Autodesk Inventor part; units mm, degrees
ref_plane "YZ Plane" through (0, 0, 0) normal (1, 0, 0) x (0, 1, 0)
ref_plane "XZ Plane" through (0, 0, 0) normal (0, 1, 0) x (-1, 0, 0)
ref_plane "XY Plane" through (0, 0, 0) normal (0, 0, 1) x (1, 0, 0)
sketch "Sketch1" plane through (0, 0, 0) normal (0, 1, 0) x (-1, 0, 0)
  circle A0 centre (0, 0) radius 165
  circle A1 centre (0, 0) radius 175
  line L0 (0, 0) -> (175, 0)
  line L1 (0, 0) -> (169.037, -45.2933)
  point P0 (159.3778, -42.7051)
  point P1 (165, 0)
  dimension "d0" = 10
  dimension "d1" = 330
  dimension "d2" = 15
extrude "Extrusion1" add sketch "Sketch1" along normal blind 5 contours L0 A1 L1 A0 picked at (171.4447, -5.0841)
sketch "Sketch3" plane through (0, 5, 0) normal (0, 1, 0) x (1, 0, 0)
  arc A0 (-169.037, 45.2933) -> (-175, 0) centre (0, 0) ccw
  line L0 (-175, 0) -> (-165, 0)
  arc A1 (-159.3778, 42.7051) -> (-165, 0) centre (0, 0) ccw
  line L1 (-159.3778, 42.7051) -> (-169.037, 45.2933)
  circle A2 centre (0, 0) radius 175
  circle A3 centre (0, 0) radius 165
  circle A4 centre (0, 0) radius 195
  line L2 (0, 0) -> (-188.3555, 50.4697)
  line L3 (0, 0) -> (-195, 0)
  point P0 (-175, 0)
  dimension "d10" = 20
extrude "Extrusion2" add sketch "Sketch3" along normal blind 10 contours L1 A1 L0 A0 | A0 L3 A4 L2
sketch "Sketch4" plane through (0, 0, 0) normal (0, -1, 0) x (1, 0, 0)
  arc A0 (-195, 0) -> (-188.3555, -50.4697) centre (0, 0) ccw
  arc A1 (-175, 0) -> (-169.037, -45.2933) centre (0, 0) ccw
  line L0 (-159.3778, -42.7051) -> (-169.037, -45.2933)
  arc A2 (-165, 0) -> (-159.3778, -42.7051) centre (0, 0) ccw
  line L1 (-175, 0) -> (-165, 0)
  circle A3 centre (0, 0) radius 175
  circle A4 centre (0, 0) radius 195
  line L2 (0, 0) -> (-175, 0)
  line L3 (0, 0) -> (-169.037, -45.2933)
  arc A5 (-175, 0) -> (-169.037, -45.2933) centre (0, 0) ccw
  line L4 (-195, 0) -> (-175, 0)
  line L5 (-169.037, -45.2933) -> (-188.3555, -50.4697)
  point P0 (-169.037, -45.2933)
extrude "Extrusion3" add sketch "Sketch4" along normal blind 10 contours L4 A1 L5 A0 | L1 A2 L0 A1
properties part number "Moving Carousel Base Inner Clip" material "PLA Plastic"
Verification items for the finished model (mm, model axes). Coordinates: 2 decimals unless noted, no trailing zeros. Loops run counter-clockwise (first coordinate to the right, second up) from the corner with the lowest first, then second, coordinate; pieces in that order, holes last. Notation, with made-up numbers: (55, -37.75) - (95, -37.75) arc R11 ccw to (95, -18.75) - close; hole circle Ø6 at (-18.75, 81). An arc over 180 degrees is marked (long way). Answer as a JSON object with one key per item and string values.
(1) Scan lines: line 1 along Y through (x, z) = (-176, -8); line 2 along Z through (x, y) = (-173, 12.5); line 3 along X through (y, z) = (-1, -19.5). Record each from-to range of solid material in increasing order.
Response:
{"line 1": "y = -10 to 0, 5 to 15", "line 2": "z = -46.36 to 0", "line 3": "x = -194.02 to -163.84"}
(2) Cross-section at A-A, the plane x = -192.5. Record the boundary of the cut face in (y, z), then the cut area to 3 significant figures.
Response:
{"outline": "(-10, -31.12) - (0, -31.12) - (0, 0) - (-10, 0) - close; (5, -31.12) - (15, -31.12) - (15, 0) - (5, 0) - close", "area": "622 mm²"}
(3) Cross-section at B-B, the plane z = -8. Record the boundary of the cut face in (x, y).
Response:
{"outline": "(-194.84, -10) - (-164.81, -10) - (-164.81, 5) - (-164.81, 15) - (-194.84, 15) - (-194.84, 5) - (-174.82, 5) - (-174.82, 0) - (-194.84, 0) - close"}
(4) Cross-section at C-C, the plane y = 9.25. Record the boundary of the cut face in (x, z), then the cut area to 3 significant figures.
Response:
{"outline": "(-195, 0) arc R195 ccw to (-188.36, -50.47) - (-169.04, -45.29) - (-159.38, -42.71) arc R165 cw to (-165, 0) - close", "area": "1,410 mm²"}
(5) Cross-section at D-D, the plane x = -185. Record the boundary of the cut face in (y, z).
Response:
{"outline": "(-10, -49.57) - (0, -49.57) - (0, 0) - (-10, 0) - close; (5, -49.57) - (15, -49.57) - (15, 0) - (5, 0) - close"}
(6) Go/stop test with flat-tipped pins: pin 1 Ø1.5 at (y, z) = (7.5, -23) entering from -X; pin 2 Ø4 at (y, z) = (7.5, -44) entering from -X; pin 3 Ø3 at (y, z) = (8.5, -6) entering from -X. Record where each tip stops, or that it passes through.
Response:
{"pin 1": "stops at x = -193.73", "pin 2": "stops at x = -190.42", "pin 3": "stops at x = -194.95"}
(7) Mould release check, pull along Y, two halves, no side actions. Record for faces 1 (the flat face through (-177, -10, -25)), 2 (the flat face through (-179.8, -0.5, 0)), 3 (the cylindrical face through (-173.544, 2.465, -22.524)): pulls with the +Y half, pulls with the -Y half, needs draft (parallel to the pull), parting line crosses it, or undercut.
Response:
{"face 1": "pulls with the -Y half", "face 2": "needs draft", "face 3": "undercut"}
